Read the model definition and answer for the solid it produces. Units are mm, in the model's axes. A direction names the side the tool comes from. Coordinates: 2 decimals unless noted, no trailing zeros. Loops run counter-clockwise (first coordinate to the right, second up) from the corner with the lowest first, then second, coordinate; pieces in that order, holes last. Notation, with made-up numbers: (66, 18.25) - (122, 18.25) arc R31 cw to (122, 47.25) - close; hole circle Ø8 at (40, 35). An arc over 180 degrees is marked (long way). Use CSV: the item, a comma, the result in double quotes.
```python
from build123d import *

# Parameters (mm, degrees)
CROQUIS1_W              = 80
CROQUIS1_H              = 60
CROQUIS1_R              = 1.5
CROQUIS1_W_2            = 7
CROQUIS1_H_2            = 25
CROQUIS1_W_3            = 10
CROQUIS1_H_3            = 20
CROQUIS1_H_4            = 10
CROQUIS1_W_4            = 5
CROQUIS1_H_5            = 6.5
SALIENTE_EXTRUIR1_DEPTH = 10
CORTAR_EXTRUIR1_DEPTH   = 5
CROQUIS3_R              = 1.5
CORTAR_EXTRUIR2_DEPTH   = 25
CROQUIS6_R              = 1.5
CORTAR_EXTRUIR3_DEPTH   = 25
CROQUIS8_W              = 15
CROQUIS8_H              = 17.838651154
CROQUIS8_R              = 1.5
SALIENTE_EXTRUIR2_DEPTH = 2
CORTAR_EXTRUIR4_START   = -55
CORTAR_EXTRUIR4_DEPTH   = 8
CROQUIS10_R             = 1.5
CROQUIS10_W             = 7
CROQUIS10_H             = 12
CORTAR_EXTRUIR5_DEPTH   = 16
CROQUIS12_W             = 110
CROQUIS12_H             = 10
SALIENTE_EXTRUIR3_DEPTH = 3
CORTAR_EXTRUIR6_DEPTH   = 5
SALIENTE_EXTRUIR4_DEPTH = 10
CROQUIS15_R             = 2.25
CORTAR_EXTRUIR7_DEPTH   = 10
CROQUIS16_R             = 2.25
CORTAR_EXTRUIR8_DEPTH   = 10


with BuildPart() as part:
    # Croquis1 → Saliente-Extruir1 (new body)
    with BuildSketch(Plane(origin=(0, 0, 0), x_dir=(1, 0, 0), z_dir=(0, 1, 0))):
        with Locations((0, -10)):
            Rectangle(CROQUIS1_W, CROQUIS1_H)
        with Locations(Location((18, -16.5, 0), (0, 0, 270))):
            Circle(CROQUIS1_R, mode=Mode.SUBTRACT)
        with Locations(Location((-11, -16.5, 0), (0, 0, 270))):
            Circle(CROQUIS1_R, mode=Mode.SUBTRACT)
        with Locations(Location((18, 16.5, 0), (0, 0, 270))):
            Circle(CROQUIS1_R, mode=Mode.SUBTRACT)
        with Locations(Location((-11, 16.5, 0), (0, 0, 270))):
            Circle(CROQUIS1_R, mode=Mode.SUBTRACT)
        with Locations((18, 0)):
            Rectangle(CROQUIS1_W_2, CROQUIS1_H_2, mode=Mode.SUBTRACT)
        Polygon((6.495190528, 3.75), (0, 7.5), (-6.495190528, 3.75), (-6.495190528, -3.75), (0, -7.5), (6.495190528, -3.75), align=None, mode=Mode.SUBTRACT)
        with Locations((-11, 0)):
            Rectangle(CROQUIS1_W_2, CROQUIS1_H_2, mode=Mode.SUBTRACT)
        with Locations((-45, -10)):
            Rectangle(CROQUIS1_W_3, CROQUIS1_H_3)
        with Locations((-45, -35)):
            Rectangle(CROQUIS1_W_3, CROQUIS1_H_4)
        with Locations((-52.5, -10)):
            Rectangle(CROQUIS1_W_4, CROQUIS1_H)
        with Locations((-45, 15)):
            Rectangle(CROQUIS1_W_3, CROQUIS1_H_4)
        with Locations((45, 15)):
            Rectangle(CROQUIS1_W_3, CROQUIS1_H_4)
        with Locations((52.5, -10)):
            Rectangle(CROQUIS1_W_4, CROQUIS1_H)
        with Locations((45, -10)):
            Rectangle(CROQUIS1_W_3, CROQUIS1_H_3)
        with Locations((45, -35)):
            Rectangle(CROQUIS1_W_3, CROQUIS1_H_4)
        with Locations((-11, 9.25)):
            Rectangle(CROQUIS1_W_2, CROQUIS1_H_5)
        with Locations((-11, -9.25)):
            Rectangle(CROQUIS1_W_2, CROQUIS1_H_5)
        with Locations((18, 9.25)):
            Rectangle(CROQUIS1_W_2, CROQUIS1_H_5)
        with Locations((18, -9.25)):
            Rectangle(CROQUIS1_W_2, CROQUIS1_H_5)
    extrude(amount=SALIENTE_EXTRUIR1_DEPTH)

    # Croquis2 → Cortar-Extruir1 (cut)
    with BuildSketch(Plane.XZ):
        Polygon((-6.958548116, 16.5), (-8.979274058, 20), (-13.020725942, 20), (-15.041451884, 16.5), (-13.020725942, 13), (-8.979274058, 13), align=None)
        Polygon((22.041451884, 16.5), (20.020725942, 20), (15.979274058, 20), (13.958548116, 16.5), (15.979274058, 13), (20.020725942, 13), align=None)
        Polygon((-6.958548116, -16.5), (-8.979274058, -13), (-13.020725942, -13), (-15.041451884, -16.5), (-13.020725942, -20), (-8.979274058, -20), align=None)
        Polygon((22.041451884, -16.5), (20.020725942, -13), (15.979274058, -13), (13.958548116, -16.5), (15.979274058, -20), (20.020725942, -20), align=None)
    extrude(amount=-CORTAR_EXTRUIR1_DEPTH, mode=Mode.SUBTRACT)

    # Croquis3 → Cortar-Extruir2 (cut)
    with BuildSketch(Plane(origin=(55, 0, 0), x_dir=(0, 0, -1), z_dir=(1, 0, 0))):
        with Locations((-25, 5)):
            Circle(CROQUIS3_R)
        with Locations((5, 5)):
            Circle(CROQUIS3_R)
    extrude(amount=-CORTAR_EXTRUIR2_DEPTH, mode=Mode.SUBTRACT)

    # Croquis6 → Cortar-Extruir3 (cut)
    with BuildSketch(Plane.ZY.offset(55)):
        with Locations(Location((-5, 5, 0), (0, 0, 180))):
            Circle(CROQUIS6_R)
        with Locations(Location((25, 5, 0), (0, 0, 180))):
            Circle(CROQUIS6_R)
    extrude(amount=-CORTAR_EXTRUIR3_DEPTH, mode=Mode.SUBTRACT)

    # Croquis8 → Saliente-Extruir2 (add)
    with BuildSketch(Plane(origin=(0, 10, 0), x_dir=(1, 0, 0), z_dir=(0, 1, 0))):
        Rectangle(CROQUIS8_W, CROQUIS8_H)
        with Locations(Location((0, 0, 0), (0, 0, 270))):
            Circle(CROQUIS8_R, mode=Mode.SUBTRACT)
    extrude(amount=-SALIENTE_EXTRUIR2_DEPTH)

    # Croquis9 → Cortar-Extruir4 (cut, symmetric)
    with BuildSketch(Plane(origin=(55, 0, 0), x_dir=(0, 0, -1), z_dir=(1, 0, 0)).offset(CORTAR_EXTRUIR4_START)):
        Polygon((-40, 3), (-12.5, 10), (-40, 10), align=None)
    extrude(amount=CORTAR_EXTRUIR4_DEPTH, both=True, mode=Mode.SUBTRACT)

    # Croquis10 → Cortar-Extruir5 (cut)
    with BuildSketch(Plane(origin=(0, 10, 0), x_dir=(1, 0, 0), z_dir=(0, 1, 0))):
        with Locations(Location((25, -12, 0), (0, 0, 270))):
            Circle(CROQUIS10_R)
        with Locations(Location((25, -36, 0), (0, 0, 270))):
            Circle(CROQUIS10_R)
        with Locations((25, -24)):
            Rectangle(CROQUIS10_W, CROQUIS10_H)
    extrude(amount=-CORTAR_EXTRUIR5_DEPTH, mode=Mode.SUBTRACT)

    # Croquis12 → Saliente-Extruir3 (add)
    with BuildSketch(Plane(origin=(0, 0, -20), x_dir=(-1, 0, 0), z_dir=(0, 0, -1))):
        with Locations((0, 5)):
            Rectangle(CROQUIS12_W, CROQUIS12_H)
    extrude(amount=SALIENTE_EXTRUIR3_DEPTH)

    # Croquis13 → Cortar-Extruir6 (cut)
    with BuildSketch(Plane.XZ):
        Polygon((29.041451884, 12), (27.020725942, 15.5), (22.979274058, 15.5), (20.958548116, 12), (22.979274058, 8.5), (27.020725942, 8.5), align=None)
        Polygon((29.041451884, 36), (27.020725942, 39.5), (22.979274058, 39.5), (20.958548116, 36), (22.979274058, 32.5), (27.020725942, 32.5), align=None)
    extrude(amount=-CORTAR_EXTRUIR6_DEPTH, mode=Mode.SUBTRACT)

    # Croquis14 → Saliente-Extruir4 (add)
    with BuildSketch(Plane.XZ):
        with BuildLine():
            Line((30, 41), (30, 42))
            ThreePointArc((30, 42), (29.707106781, 42.707106781), (29, 43))
            Line((29, 43), (21, 43))
            ThreePointArc((21, 43), (20.292893219, 42.707106781), (20, 42))
            Line((20, 42), (20, 41))
            ThreePointArc((20, 41), (19.707106781, 40.292893219), (19, 40))
            Line((19, 40), (31, 40))
            ThreePointArc((31, 40), (30.292893219, 40.292893219), (30, 41))
        make_face()
    extrude(amount=-SALIENTE_EXTRUIR4_DEPTH)

    # Croquis15 → Cortar-Extruir7 (cut)
    with BuildSketch(Plane(origin=(55, 0, 0), x_dir=(0, 0, -1), z_dir=(1, 0, 0))):
        with Locations((-25, 5)):
            Circle(CROQUIS15_R)
        with Locations((5, 5)):
            Circle(CROQUIS15_R)
    extrude(amount=-CORTAR_EXTRUIR7_DEPTH, mode=Mode.SUBTRACT)

    # Croquis16 → Cortar-Extruir8 (cut)
    with BuildSketch(Plane.ZY.offset(55)):
        with Locations(Location((-5, 5, 0), (0, 0, 180))):
            Circle(CROQUIS16_R)
        with Locations(Location((25, 5, 0), (0, 0, 180))):
            Circle(CROQUIS16_R)
    extrude(amount=-CORTAR_EXTRUIR8_DEPTH, mode=Mode.SUBTRACT)


solid = part.part
```
Q1. A tool of negligible diameter and unlimited length cuts with its end or side. For faces 1 (the face through (-7.5, 5, 0)), 2 (the face through (0.11, 6.45, 26.44)), 3 (the face through (-9, 5, 17)), from which of +Z, -Z, +X, -X, +Y, -Y can it reach the whole face along a straight path? Write none if from no direction.
Reported:
face 1,"+Y, -Y"
face 2,"+Z, +Y"
face 3,"-Y"
Q2. The part is cut by section A-A on x = 25. Determine the outline of the cut face in (y, z).
Reported:
outline,"(0, -23) - (10, -23) - (10, 10.5) - (5, 10.5) - (5, 8.5) - (0, 8.5) - close; (0, 15.5) - (5, 15.5) - (5, 13.5) - (10, 13.5) - (10, 18) - (0, 18) - close; (0, 30) - (10, 30) - (10, 34.5) - (5, 34.5) - (5, 32.5) - (0, 32.5) - close; (0, 39.5) - (5, 39.5) - (5, 37.5) - (10, 37.5) - (10, 43) - (0, 43) - close"
Q3. Find the intervals of material crossed by probe 1 along X at (y, z) = (0.75, -3); probe 2 along X at (y, z) = (7, 16.5); probe 3 along Z at (x, y) = (47, 5), in increasing order. Write a range as [from, to].
Reported:
probe 1,"x = [-55, -50], [-40, -14.5], [-7.5, -6.5], [6.5, 14.5], [21.5, 40], [50, 55]"
probe 2,"x = [-55, -12.5], [-9.5, 16.5], [19.5, 55]"
probe 3,"z = [-23, -10], [0, 20], [30, 40]"
Q4. Given P1, Ø5, axis at x = 6, y = 2.5, coming from the +Z side; P2, Ø0.5, axis at y = 4, z = 41.5, coming from the -X side; P3, Ø5, axis at x = 38, z = 31.5, coming from the -Y side; P4, Ø5, axis at x = -11, z = 16.5, coming from the -Y side, each flat-ended and moving along its own axis, determine where each tip first touches the part or whether it passes through.
Reported:
P1,"stops at z = 40"
P2,"stops at x = 20"
P3,"stops at y = 0"
P4,"stops at y = 5"
Q5. The part is cut by section B-B on x = -23. Determine the outline of the cut face in (y, z), and give its area (3 significant figures).
Reported:
outline,"(0, -23) - (10, -23) - (10, 40) - (0, 40) - close"
area,"630 mm²"
Q6. The part is cut by section C-C on z = 25. Give the number of separate pieces and of enclosed holes in the cut face, and give its area (3 significant figures).
Reported:
separate pieces,"6"
enclosed holes,"0"
area,"674 mm²"
Q7. For a pull along X with two mould halves and no side action, classify faces 4 (the face through (1, 5, -23)), 5 (the face through (-11, 2, 13)) as +X half, -X half, draft (parallel to the pull), parting line (faces both ways), or undercut.
Reported:
face 4,"draft"
face 5,"undercut"
